from build123d import *

# Parameters (mm, degrees)
SKETCH1_R           = 1.25
BOSS_EXTRUDE1_DEPTH = 3.9
BOSS_EXTRUDE2_DEPTH = 8
SKETCH4_R           = 1.25
CUT_EXTRUDE1_DEPTH  = 4.8
SKETCH5_OUTSIDE_W   = 35.048
SKETCH5_OUTSIDE_H   = 35.744
SKETCH5_OUTSIDE_R   = 2.257033445
CUT_EXTRUDE2_DEPTH  = 12.9
CUT_EXTRUDE2_TAPER  = 45
SKETCH6_OUTSIDE_W   = 27.248
SKETCH6_OUTSIDE_H   = 27.944
SKETCH6_OUTSIDE_R   = 2.25
CUT_EXTRUDE3_DEPTH  = 9
CUT_EXTRUDE3_TAPER  = 45
CHAMFER1_SIZE       = 0.3
CHAMFER1_SIZE2      = 0.357526078


with BuildPart() as part:
    # Sketch1 → Boss-Extrude1 (new body)
    with BuildSketch(Plane(origin=(0, 0, 0), x_dir=(1, 0, 0), z_dir=(0, 1, 0))):
        Circle(SKETCH1_R)
    extrude(amount=BOSS_EXTRUDE1_DEPTH)

    # Sketch3 → Boss-Extrude2 (add)
    with BuildSketch(Plane(origin=(0, 3.9, 0), x_dir=(1, 0, 0), z_dir=(0, 1, 0))):
        Polygon((-2.25, 1.299038106), (-2.25, -1.299038106), (0, -2.598076211), (2.25, -1.299038106), (2.25, 1.299038106), (0, 2.598076211), align=None)
    extrude(amount=BOSS_EXTRUDE2_DEPTH)

    # Sketch4 → Cut-Extrude1 (cut)
    with BuildSketch(Plane(origin=(0, 11.9, 0), x_dir=(1, 0, 0), z_dir=(0, 1, 0))):
        Circle(SKETCH4_R)
    extrude(amount=-CUT_EXTRUDE1_DEPTH, mode=Mode.SUBTRACT)

    # Sketch5 outside → Cut-Extrude2 (cut, through all)
    with BuildSketch(Plane(origin=(0, 11.9, 0), x_dir=(1, 0, 0), z_dir=(0, 1, 0))):
        Rectangle(SKETCH5_OUTSIDE_W, SKETCH5_OUTSIDE_H)
        Circle(SKETCH5_OUTSIDE_R, mode=Mode.SUBTRACT)
    extrude(amount=-CUT_EXTRUDE2_DEPTH, taper=CUT_EXTRUDE2_TAPER, mode=Mode.SUBTRACT)

    # Sketch6 outside → Cut-Extrude3 (cut, through all)
    with BuildSketch(Plane.XZ.offset(-3.9)):
        Rectangle(SKETCH6_OUTSIDE_W, SKETCH6_OUTSIDE_H)
        Circle(SKETCH6_OUTSIDE_R, mode=Mode.SUBTRACT)
    extrude(amount=-CUT_EXTRUDE3_DEPTH, taper=CUT_EXTRUDE3_TAPER, mode=Mode.SUBTRACT)

    # Chamfer1
    chamfer1_edges = [part.edges().sort_by_distance(p)[0] for p in [
        (-1.25, 0, 0),
    ]]
    chamfer1_side = [part.faces().sort_by_distance(p)[0] for p in [
        (0, 0, 0),
    ]]
    chamfer(chamfer1_edges, length=CHAMFER1_SIZE, length2=CHAMFER1_SIZE2, reference=chamfer1_side[0])


solid = part.part
Read the model definition and answer for the solid it produces. Units are mm, in the model's axes. A direction names the side the tool comes from. Round coordinates to 2 decimals unless told otherwise and drop trailing zeros. Write each loop counter-clockwise with the first axis right and the second up, starting at its lowest first coordinate (ties: lowest second). Pieces come first, ordered by that corner, then holes. Notation, with made-up numbers: (35, 76.25) - (86, 76.25) arc R10 ccw to (86, 87.25) - close; hole circle Ø10 at (82.5, 4.25). An arc over 180 degrees is marked (long way). Use a Markdown table: item, result.
(1) Each of these flat-tipped pins is pushed along its axis until it touches: pin 1 Ø3 at (y, z) = (4, -1.5) entering from -X; pin 2 Ø1.2 at (x, z) = (0, 0.5) entering from +Y. Where does it stop, or does it pass through?
Reported:
| item | result |
|---|---|
| pin 1 | x = -2.25 |
| pin 2 | y = 7.1 |
(2) Which of the six approach directions +Z, -Z, +X, -X, +Y, -Y give full straight-line access (tool end or side, diameter ignored) to faces 1 (the conical face through (-2.06, 11.78, 1.19)), 2 (the flat face through (1, 3.9, 1)), 3 (the flat face through (0, 7.1, 0))?
Reported:
| item | result |
|---|---|
| face 1 | +Z, -X, +Y |
| face 2 | -Y |
| face 3 | +Y |
(3) The part is cut by section B-B (y = 1.75). Write down the section's boundary in (x, z), then the cut area to 3 significant figures.
Reported:
| item | result |
|---|---|
| outline | circle Ø2.5 at (0, 0) |
| area | 4.91 mm2 |
(4) The part is cut by section A-A (y = 7.5). Write down the section's boundary in (x, z).
Reported:
| item | result |
|---|---|
| outline | (-2.25, -1.3) - (0, -2.6) - (2.25, -1.3) - (2.25, 1.3) - (0, 2.6) - (-2.25, 1.3) - close; hole circle Ø2.5 at (0, 0) |
(5) Straight lines are drawn through the part: line 1 along X through (y, z) = (8.55, 0); line 2 along Y through (x, z) = (1.6, 1.5); line 3 along Z through (x, y) = (-0.95, 10). For each, find the intervals that lie inside material, in ascending order. Write a range as [from, to].
Reported:
| item | result |
|---|---|
| line 1 | [-2.25, -1.25], [1.25, 2.25] |
| line 2 | [3.9, 11.9] |
| line 3 | [-2.05, -0.81], [0.81, 2.05] |
(6) The mould has two halves that part along Z. Classify faces 4 (the conical face through (2.05, 4.02, 1.19)), 5 (the flat face through (2.25, 8, 0)), 6 (the cylindrical face through (-0.27, 9.53, 1.22)): released by +Z, released by -Z, zero draft, split by the parting line, or undercut.
Reported:
| item | result |
|---|---|
| face 4 | released by +Z |
| face 5 | zero draft |
| face 6 | undercut |
